Could you check a few things on this model? Use its own coordinates, in mm. A direction names the side the tool comes from. Coordinates: 2 decimals unless noted, no trailing zeros. Write each loop counter-clockwise with the first axis right and the second up, starting at its lowest first coordinate (ties: lowest second). Pieces come first, ordered by that corner, then holes.
```python
from build123d import *

# Parameters (mm, degrees)
SKETCH1_W            = 34
SKETCH1_H            = 37
SKETCH1_R            = 2.7
BOSS_EXTRUDE1_DEPTH  = 4
SKETCH30_W           = 37
SKETCH30_H           = 25
BOSS_EXTRUDE19_DEPTH = 3
SKETCH31_W           = 37
SKETCH31_H           = 25
BOSS_EXTRUDE20_DEPTH = 3


with BuildPart() as part:
    # Sketch1 → Boss-Extrude1 (new body)
    with BuildSketch(Plane(origin=(0, 0, 0), x_dir=(1, 0, 0), z_dir=(0, 1, 0))):
        with Locations((-18.825390803, 9.424231459)):
            Rectangle(SKETCH1_W, SKETCH1_H)
        with Locations(Location((-18.825390803, 20.924231459, 0), (0, 0, 270))):
            Circle(SKETCH1_R, mode=Mode.SUBTRACT)
        with Locations(Location((-11.325390803, 0.924231459, 0), (0, 0, 270))):
            Circle(SKETCH1_R, mode=Mode.SUBTRACT)
        with Locations(Location((-26.325390803, 0.924231459, 0), (0, 0, 90))):
            Circle(SKETCH1_R, mode=Mode.SUBTRACT)
    extrude(amount=BOSS_EXTRUDE1_DEPTH)

    # Sketch30 → Boss-Extrude19 (add)
    with BuildSketch(Plane.ZY.offset(35.825390803)):
        with Locations((-9.424231459, 16.5)):
            Rectangle(SKETCH30_W, SKETCH30_H)
    extrude(amount=-BOSS_EXTRUDE19_DEPTH)

    # Sketch31 → Boss-Extrude20 (add)
    with BuildSketch(Plane(origin=(-1.825390803, 0, 0), x_dir=(0, 0, -1), z_dir=(1, 0, 0))):
        with Locations((9.424231459, 16.5)):
            Rectangle(SKETCH31_W, SKETCH31_H)
    extrude(amount=-BOSS_EXTRUDE20_DEPTH)


solid = part.part
```
1. On a 3-axis mill with a long thin cutter (end or side, diameter ignored), from which of +Z, -Z, +X, -X, +Y, -Y can I reach the whole of each face in a straight line? I mean faces 4 (the face through (-19, 0, -10)), 5 (the face through (-19, 4, -10)). Say none if no direction works.
Verdict:
face 4: +Z, -Z, +X, -X, -Y
face 5: +Z, -Z, +Y
2. I want a section at A-A on y = 20.5. Please give me the cut outline in (x, z).
Verdict:
outline: (-35.83, -27.92) - (-32.83, -27.92) - (-32.83, 9.08) - (-35.83, 9.08) - close; (-4.83, -27.92) - (-1.83, -27.92) - (-1.83, 9.08) - (-4.83, 9.08) - close
3. Please list where these lines run through material, in increasing order: line 1 along X through (y, z) = (11.5, 3); line 2 along Y through (x, z) = (-13, -3.5); line 3 along X through (y, z) = (2.25, -2.5).
Verdict:
line 1: x = -35.83 to -32.83, -4.83 to -1.83
line 2: y = 0 to 4
line 3: x = -35.83 to -28.52, -24.13 to -13.52, -9.13 to -1.83
4. I want a section at C-C on x = -25. Please give me the cut outline in (y, z), plus the area to 3 significant figures.
Verdict:
outline: (0, -27.92) - (4, -27.92) - (4, -3.28) - (0, -3.28) - close; (0, 1.43) - (4, 1.43) - (4, 9.08) - (0, 9.08) - close
area: 129 mm2
5. For pin 1 (6 mm diameter, centred on x = -26.33, z = -0.92, fed in from +Y), with a flat end and sliding along its axis, tell me the tip position at first contact or that it passes through.
Verdict:
pin 1: stops at y = 4
6. I want a section at D-D on z = -24.5. Please give me the cut outline in (x, y), plus the area to 3 significant figures.
Verdict:
outline: (-35.83, 0) - (-1.83, 0) - (-1.83, 29) - (-4.83, 29) - (-4.83, 4) - (-32.83, 4) - (-32.83, 29) - (-35.83, 29) - close
area: 286 mm2
7. I want a section at B-B on z = 1. Please give me the cut outline in (x, y).
Verdict:
outline: (-35.83, 0) - (-28.22, 0) - (-28.22, 4) - (-32.83, 4) - (-32.83, 29) - (-35.83, 29) - close; (-24.43, 0) - (-13.22, 0) - (-13.22, 4) - (-24.43, 4) - close; (-9.43, 0) - (-1.83, 0) - (-1.83, 29) - (-4.83, 29) - (-4.83, 4) - (-9.43, 4) - close
8. If we mould it in two halves opening along X, with no side actions, what happens to faces 1 (the face through (-35.825, 15, -10)), 2 (the face through (-13.72, 1.97, 0.32)), 3 (the face through (-20, 3.7, -27.924))? For each: pulls with the +X half, pulls with the -X half, needs draft (parallel to the pull), parting line crosses it, or undercut.
Verdict:
face 1: pulls with the -X half
face 2: undercut
face 3: needs draft
